Build history of the part. All positions in model axes, mm. A direction names the side the tool comes from. Give positions to 0.01 mm unless a question says otherwise; leave off trailing zeros. Order: outer loops, then holes, each group sorted by start corner. A loop starts at its lowest first (then second) coordinate and runs counter-clockwise, first axis right, second up. Notation, with made-up numbers: M 41.5,2.5 L 45.5,2.5 A14 cw 45.5,13.5 Z; hole C -19,65 d8. An arc over 180 degrees is marked long. One line per item, written item: value.
from build123d import *

# Parameters (mm, degrees)
BOSS_EXTRU_1_OUTLINE_W   = 5
BOSS_EXTRU_1_OUTLINE_H   = 5
BOSS_EXTRU_1_OUTLINE_R   = 1.5
BOSS_EXTRU_1_OUTLINE_R_2 = 1.25
BOSS_EXTRU_1_DEPTH       = 5
CONG_1_R                 = 5


# Read off the part's stored shape, not the designer's step: Boss.-Extru.1
with BuildPart() as part:
    # Boss.-Extru.1 outline → Boss.-Extru.1 (new body)
    with BuildSketch(Plane.XY):
        Polygon((47.6, 5.3), (47.6, 3), (46.5, 3), (46.5, 0), (50, 0), (50, -5), (55, -5), (55, 0), (105, 0), (105, -5), (110, -5), (110, 0), (113.5, 0), (113.5, 3), (112.4, 3), (112.4, 5.3), (113.5, 5.3), (113.5, 10), (116.5, 10), (116.5, 5.3), (117.6, 5.3), (117.6, 3), (116.5, 3), (116.5, 0), (120, 0), (120, -5), (125, -5), (125, 0), (175, 0), (175, -5), (180, -5), (180, 0), (183.5, 0), (183.5, 3), (182.4, 3), (182.4, 5.3), (183.5, 5.3), (183.5, 10), (186.5, 10), (186.5, 5.3), (187.6, 5.3), (187.6, 3), (186.5, 3), (186.5, 0), (190, 0), (190, -5), (195, -5), (195, 0), (230, 0), (230, 40), (0, 40), (0, 0), (35, 0), (35, -5), (40, -5), (40, 0), (43.5, 0), (43.5, 3), (42.4, 3), (42.4, 5.3), (43.5, 5.3), (43.5, 10), (46.5, 10), (46.5, 5.3), align=None)
        with Locations((7.5, 7.5)):
            Rectangle(BOSS_EXTRU_1_OUTLINE_W, BOSS_EXTRU_1_OUTLINE_H, mode=Mode.SUBTRACT)
        with Locations((7.5, 15)):
            Circle(BOSS_EXTRU_1_OUTLINE_R, mode=Mode.SUBTRACT)
        with Locations((222.5, 7.5)):
            Rectangle(BOSS_EXTRU_1_OUTLINE_W, BOSS_EXTRU_1_OUTLINE_H, mode=Mode.SUBTRACT)
        with Locations((222.5, 15)):
            Circle(BOSS_EXTRU_1_OUTLINE_R, mode=Mode.SUBTRACT)
        with Locations((7.5, 22.5)):
            Rectangle(BOSS_EXTRU_1_OUTLINE_W, BOSS_EXTRU_1_OUTLINE_H, mode=Mode.SUBTRACT)
        with Locations((91, 18)):
            Circle(BOSS_EXTRU_1_OUTLINE_R_2, mode=Mode.SUBTRACT)
        with Locations((117, 18)):
            Circle(BOSS_EXTRU_1_OUTLINE_R_2, mode=Mode.SUBTRACT)
        with Locations((222.5, 22.5)):
            Rectangle(BOSS_EXTRU_1_OUTLINE_W, BOSS_EXTRU_1_OUTLINE_H, mode=Mode.SUBTRACT)
    extrude(amount=BOSS_EXTRU_1_DEPTH)

    # Congé1
    cong_1_edges = [part.edges().sort_by_distance(p)[0] for p in [
        (0, 0, 2.5),
        (0, 40, 2.5),
        (230, 40, 2.5),
        (230, 0, 2.5),
    ]]
    fillet(cong_1_edges, radius=CONG_1_R)


solid = part.part
1) Mould opens along X. For faces 4 (the face through (5, 22, 2)), 5 (the face through (228, 39, 3)), 6 (the face through (37, -5, 2)) say: released by +X, released by -X, zero draft, split by the parting line, or undercut.
Check values:
face 4: undercut
face 5: released by +X
face 6: zero draft
2) Drill centre lines: probe 1 along X at (y, z) = (8.5, 2); probe 2 along X at (y, z) = (24, 1.8); probe 3 along Y at (x, z) = (222.5, 3.1). Where is each one in solid material? Low to high. Write a range as from..to.
Check values:
probe 1: 0..5, 10..43.5, 46.5..113.5, 116.5..183.5, 186.5..220, 225..230
probe 2: 0..5, 10..220, 225..230
probe 3: 0..5, 10..13.5, 16.5..20, 25..40
3) Saw through at A-A, the plane z = 2.05. Give the number of separate pieces and of enclosed holes in the cut face, then the cut area to 3 significant figures.
Check values:
separate pieces: 1
enclosed holes: 8
area: 9,100 mm^2
4) Pin check, flat tips, straight feed: pin 1 (2.5 mm diameter, centred on y = 2, z = 2, fed in from -X); pin 2 (1.2 mm diameter, centred on y = 4, z = 3, fed in from +X); pin 3 (1.8 mm diameter, centred on y = 4, z = 2, fed in from -X); pin 4 (1 mm diameter, centred on x = 181.5, z = 3, fed in from -Y). Stop position of each tip, or through.
Check values:
pin 1: x = 0.32
pin 2: x = 229.98
pin 3: x = 0
pin 4: y = 0
5) Tool access for faces 1 (the face through (186.5, 8, 2)), 2 (the face through (210, 0, 2)), 3 (the face through (225, 22, 2)): list every direction of +Z, -Z, +X, -X, +Y, -Y with a clear straight run to the whole face (end or side of a thin tool).
Check values:
face 1: +Z, -Z, -Y
face 2: +Z, -Z, +X, -Y
face 3: +Z, -Z
6) Saw through at B-B, the plane x = 139. Write the cut outline in (y, z), then the cut area to 3 significant figures.
Check values:
outline: M 0,0 L 40,0 L 40,5 L 0,5 Z
area: 200 mm^2
